from build123d import *

# Parameters (mm, degrees)
ESQUISSE1_R             = 320
BOSS_EXTRU_1_DEPTH      = 200
CHANFREIN2_SIZE         = 70
ESQUISSE2_R             = 320
ESQUISSE2_R_2           = 317
BOSS_EXTRU_2_DEPTH      = 180
ESQUISSE3_W             = 440
ESQUISSE3_H             = 180
ENL_V_MAT_EXTRU_1_DEPTH = 591.931468108


with BuildPart() as part:
    # Esquisse1 → Boss.-Extru.1 (new body)
    with BuildSketch(Plane.XY):
        Circle(ESQUISSE1_R)
    extrude(amount=BOSS_EXTRU_1_DEPTH)

    # Chanfrein2
    chanfrein2_edges = [part.edges().sort_by_distance(p)[0] for p in [
        (-320, 0, 0),
    ]]
    chamfer(chanfrein2_edges, length=CHANFREIN2_SIZE)

    # Esquisse2 → Boss.-Extru.2 (add)
    with BuildSketch(Plane.XY.offset(200)):
        Circle(ESQUISSE2_R)
        with Locations(Location((0, 0, 0), (0, 0, 180))):
            Circle(ESQUISSE2_R_2, mode=Mode.SUBTRACT)
    extrude(amount=BOSS_EXTRU_2_DEPTH)

    # Esquisse3 → Enlèv. mat.-Extru.1 (cut, through all)
    with BuildSketch(Plane(origin=(0, 0, 0), x_dir=(1, 0, 0), z_dir=(0, 1, 0))):
        with Locations((0, -290)):
            Rectangle(ESQUISSE3_W, ESQUISSE3_H)
    extrude(amount=-ENL_V_MAT_EXTRU_1_DEPTH, mode=Mode.SUBTRACT)


solid = part.part
The listing builds one solid part. Answer for the finished solid, in the listing's coordinates (mm). Give positions to 0.01 mm unless a question says otherwise; leave off trailing zeros. Write each loop counter-clockwise with the first axis right and the second up, starting at its lowest first coordinate (ties: lowest second). Pieces come first, ordered by that corner, then holes.
Item 1: Flat-ended cylindrical pins translate along their axes: P1, Ø2, axis at y = -230, z = 296.5, coming from the +X side; P2, Ø2, axis at x = 50.5, z = 244, coming from the +Y side; P3, Ø4, axis at y = -21.5, z = 282, coming from the -X side. Find the tip coordinate at first contact, or state that the pin passes through.
Item 2: Section D-D, the plane z = 341 is taken. Write down the section's boundary in (x, y).
Item 3: Determine the mould class of faces 1 (the flat face through (-3, 3, 0)), 2 (the cylindrical face through (-41.658, 317.277, 222.83)), 3 (the cylindrical face through (10.536, 316.825, 288.74)), 4 (the flat face through (-4, 3, 200)) for opening direction X: released by +X, released by -X, zero draft, split by the parting line, or undercut.
Item 4: Section C-C, the plane z = 79 is taken. Write down the section's boundary in (x, y).
Item 5: Section B-B, the plane y = 0 is taken. Write down the section's boundary in (x, z).
Item 6: Section A-A, the plane x = 0 is taken. Write down the section's boundary in (y, z), plus the area to 3 significant figures.
Item 7: Find the intervals of material crossed by line 1 along X through (y, z) = (0, 325); line 2 along Y through (x, z) = (0, 295); line 3 along Z through (x, y) = (-127, -61.5), in increasing order.
Completed:
1. P1: stops at x = 223.52
1. P2: stops at y = 316.15
1. P3: stops at x = -319.41
2. outline: (-220, -232.38) - (-220, -228.23) arc R317 cw (long way) to (220, -228.23) - (220, -232.38) arc R320 ccw (long way) to start
3. face 1: zero draft
3. face 2: split by the parting line
3. face 3: undercut
3. face 4: undercut
4. outline: circle Ø640 at (0, 0)
5. outline: (-320, 70) - (-250, 0) - (250, 0) - (320, 70) - (320, 380) - (317, 380) - (317, 200) - (-317, 200) - (-317, 380) - (-320, 380) - close
6. outline: (-320, 70) - (-250, 0) - (250, 0) - (320, 70) - (320, 380) - (317, 380) - (317, 200) - (-320, 200) - close
6. area: 124,000 mm2
7. line 1: x = -320 to -317, 317 to 320
7. line 2: y = 317 to 320
7. line 3: z = 0 to 200
